For this review, take the finished solid that the model builds, in its own axes (mm). A direction names the side the tool comes from. Coordinates: 2 decimals unless noted, no trailing zeros. Write each loop counter-clockwise with the first axis right and the second up, starting at its lowest first coordinate (ties: lowest second). Pieces come first, ordered by that corner, then holes. Notation, with made-up numbers: (37, 66.25) -> (88, 66.25) arc R14 cw to (88, 76.25) -> close; hole circle Ø11 at (49.25, 12.25). An arc over 180 degrees is marked (long way). One line per item, written item: value. Start each with the question number.
1) Add section D-D (x = -8). State the section outline as (y, z) points, and give its area (3 significant figures).
2) For pin 1 Ø5.5 at (y, z) = (1.5, -4) entering from -X; pin 2 Ø12 at (y, z) = (12, -13.5) entering from +X; pin 3 Ø6 at (x, z) = (-8, -1.9) entering from +Y; pin 4 Ø5 at (x, y) = (-23.75, 15) entering from -Z, all flat-tipped, find the tip position at first contact; note any pin that passes through.
3) Mouldability with a two-part tool opening along Z and no side actions: class faces 4 (the flat face through (-10, 25, 14)), 5 (the cylindrical face through (5.77, 2.54, -17.6)), 6 (the flat face through (0, 2, -23.646)) as released by +Z, released by -Z, zero draft, split by the parting line, or undercut.
4) Machinability: for faces 1 (the flat face through (0, 5, -10)), 2 (the flat face through (13.75, 10, 10)), 3 (the flat face through (-13.75, 2, -10)), which of the approach directions +Z, -Z, +X, -X, +Y, -Y give a long, thin tool a straight path to every point of the face, cutting with its end or side? Answer none if there is none.
5) Add section A-A (x = -23.75). State the section outline as (y, z) points.
6) For probe 1 along X at (y, z) = (15, 9); probe 2 along Z at (x, y) = (8, 1); probe 3 along Y at (x, z) = (-23.75, 16.5), list the stretches that pass through material, from the lowest coordinate up. Write a range as from..to.
7) Add section B-B (y = 3.5). State the section outline as (x, z) points, and give its area (3 significant figures).
8) Add section C-C (y = 15). State the section outline as (x, z) points.
Autodesk Inventor part; units mm, degrees
ref_plane "YZ Plane" through (0, 0, 0) normal (1, 0, 0) x (0, 1, 0)
ref_plane "XZ Plane" through (0, 0, 0) normal (0, 1, 0) x (-1, 0, 0)
ref_plane "XY Plane" through (0, 0, 0) normal (0, 0, 1) x (1, 0, 0)
sketch "Sketch1" plane through (0, 0, 0) normal (0, 1, 0) x (-1, 0, 0)
  line L0 (-13.75, 23.6455) -> (13.75, 23.6455)
  line L1 (13.75, 23.6455) -> (13.75, -23.6455)
  line L2 (13.75, -23.6455) -> (-13.75, -23.6455)
  line L3 (-13.75, -23.6455) -> (-13.75, 23.6455)
  line L4 (-13.75, 23.6455) -> (13.75, -23.6455) construction
  line L5 (13.75, 23.6455) -> (-13.75, -23.6455) construction
  point P0 (0, 0)
  dimension "d0" = 47.291
  dimension "d1" = 27.5
extrude "Extrusion1" add sketch "Sketch1" along normal blind 5
sketch "Sketch2" plane through (0, 5, 0) normal (0, 1, 0) x (1, 0, 0)
  line L0 (-13.75, 23.6455) -> (-13.75, -23.6455)
  line L1 (13.75, -23.6455) -> (13.75, 23.6455)
  line L2 (-13.75, -23.6455) -> (13.75, -23.6455)
  line L3 (13.75, -23.6455) -> (13.75, -3.8545)
  line L4 (13.75, -3.8545) -> (-13.75, -3.8545)
  line L5 (-13.75, -3.8545) -> (-13.75, -23.6455)
  point P0 (0, 0)
  dimension "d4" = 19.791
extrude "Extrusion2" add sketch "Sketch2" along normal blind 20
sketch "Sketch5" plane through (-13.75, 0, -23.6455) normal (-1, 0, 0) x (0, 0, 1)
  line L0 (47.291, 25) -> (27.5, 25)
  line L1 (0, 0) -> (47.291, 0)
  line L2 (47.291, 25) -> (27.5, 25)
  line L3 (27.5, 25) -> (27.5, 0)
  line L4 (27.5, 0) -> (47.291, 0)
  line L5 (47.291, 0) -> (47.291, 25)
  line L6 (27.5, 5) -> (27.5, 25)
  point P0 (23.6455, 0)
  dimension "d27" = 0
extrude "Extrusion3" add sketch "Sketch5" along normal blind 20
sketch "Sketch3" plane through (0, 0, 0) normal (0, -1, 0) x (1, 0, 0)
  line L0 (13.75, -23.6455) -> (-13.75, -23.6455)
  line L1 (13.75, 23.6455) -> (13.75, -23.6455)
  point P0 (0, 0)
  point P1 (8, -17.8955)
  point P2 (-8, -1.8955)
  dimension "d7" = 5.75
  dimension "d8" = 5.75
  dimension "d9" = 16
  dimension "d10" = 16
hole "Hole1" at (8, 0, -17.8955) at (-8, 0, -1.8955) direction (0, 1, 0) diameter 4.5 end through all
sketch "Sketch4" plane through (13.75, 5, 3.8545) normal (0, 0, -1) x (-1, 0, 0)
  line L0 (27.5, 0) -> (27.5, 20)
  line L1 (27.5, 0) -> (0, 0)
  line L2 (47.5, 20) -> (47.5, -5)
  point P0 (13.75, -5)
  point P1 (37.5, 10)
  dimension "d19" = 10
  dimension "d30" = 10
hole "Hole2" at (-23.75, 15, 3.8545) direction (0, 0, 1) diameter 4.134 end through all
properties part number "ER_Positionierungseinheit_Greifer"
Numbers:
1. outline: (0, -23.65) -> (5, -23.65) -> (5, -4.15) -> (0, -4.15) -> close; (0, 0.35) -> (5, 0.35) -> (5, 3.85) -> (25, 3.85) -> (25, 23.65) -> (0, 23.65) -> close
1. area: 610 mm²
2. pin 1: x = -13.75
2. pin 2: through
2. pin 3: y = 5
2. pin 4: z = 3.85
3. face 4: zero draft
3. face 5: undercut
3. face 6: released by -Z
4. face 1: -Z, +X, -X, +Y
4. face 2: +Z, -Z, +X, +Y, -Y
4. face 3: -Z, -X, +Y, -Y
5. outline: (0, 3.85) -> (12.93, 3.85) -> (12.93, 23.65) -> (0, 23.65) -> close; (17.07, 3.85) -> (25, 3.85) -> (25, 23.65) -> (17.07, 23.65) -> close
6. probe 1: -33.75..-25.82, -21.68..13.75
6. probe 2: -23.65..-20.15, -15.65..23.65
6. probe 3: 0..12.93, 17.07..25
7. outline: (-33.75, 3.85) -> (-13.75, 3.85) -> (-13.75, -23.65) -> (13.75, -23.65) -> (13.75, 23.65) -> (-33.75, 23.65) -> close; hole circle Ø4.5 at (-8, -1.9); hole circle Ø4.5 at (8, -17.9)
7. area: 1,660 mm²
8. outline: (-33.75, 3.85) -> (-25.82, 3.85) -> (-25.82, 23.65) -> (-33.75, 23.65) -> close; (-21.68, 3.85) -> (13.75, 3.85) -> (13.75, 23.65) -> (-21.68, 23.65) -> close
